Autodesk Inventor part; units mm, degrees
ref_plane "YZ Plane" through (0, 0, 0) normal (1, 0, 0) x (0, 1, 0)
ref_plane "XZ Plane" through (0, 0, 0) normal (0, 1, 0) x (-1, 0, 0)
ref_plane "XY Plane" through (0, 0, 0) normal (0, 0, 1) x (1, 0, 0)
sketch "Sketch1" plane through (0, 0, 0) normal (0, 1, 0) x (-1, 0, 0)
  line L0 (-9, -9) -> (-9, 9)
  line L1 (-9, 9) -> (9, 9)
  line L2 (-8, -8) -> (-8, 8)
  line L3 (-8, 8) -> (8, 8)
  line L4 (0, -8) -> (0, -9)
  line L5 (0, -9) -> (-1, -9)
  line L6 (-8, -8) -> (0, -8)
  line L7 (-9, -9) -> (0, -9)
  line L8 (9, 0) -> (9, 9)
  line L9 (8, 8) -> (8, 1)
  line L10 (9, 0) -> (8, 0)
  line L11 (8, 0) -> (8, 1.1953)
  line L12 (8, 8) -> (8, 9)
  line L13 (-8, 8) -> (-8, 9)
  line L14 (9, 9) -> (8, 9)
  line L15 (-8, 9) -> (-9, 9)
  line L16 (8, 8) -> (7, 8)
  line L17 (7, 8) -> (7, 9)
  line L18 (-8, 8) -> (-7, 8)
  line L19 (-7, 9) -> (-8, 9)
  line L20 (-8, 8) -> (-7, 8)
  line L21 (-7, 8) -> (-7, 9)
  point P0 (0, 0)
  point P1 (0, 11.1675)
  dimension "d4" = 18
  dimension "d5" = 18
  dimension "d10" = 16
  dimension "d11" = 16
  dimension "d33" = 1
  dimension "d62" = 1
  dimension "d63" = 1
extrude "Extrusion1" add sketch "Sketch1" against normal blind 1 contours L0 L1 L13 L2 L6 L4 L5 L7 | L1 L21 L3 L13 | L1 L12 L3 L17 | L1 L8 L10 L11 L9 L12
ref_plane "Work Plane1" through (0, -12, 0) normal (0, -1, 0) x (1, 0, 0)
ref_plane "Work Plane6" through (0, -1, 0) normal (0, -1, 0) x (1, 0, 0)
sketch "Sketch11" plane through (0, -1, 0) normal (0, -1, 0) x (1, 0, 0)
  line L0 (9, 9) -> (-9, 9)
  line L1 (-9, 9) -> (-9, 7)
  line L2 (-9, 0) -> (-9, 9)
  line L3 (-8, 0) -> (-8, 8)
  line L4 (-8, 8) -> (8, 8)
  line L5 (-8, 7) -> (-8, 8)
  line L6 (-8, 8) -> (-7, 8)
  line L7 (-7, 8) -> (-7, 9)
  line L8 (-7, 9) -> (-9, 9)
  line L9 (-9, 7) -> (-8, 7)
  line L10 (9, -9) -> (9, 9)
  line L11 (9, 9) -> (7, 9)
  line L12 (7, 9) -> (7, 8)
  line L13 (7, 8) -> (8, 8)
  line L14 (8, 8) -> (8, 7)
  line L15 (8, 8) -> (8, -8)
  line L16 (9, 7) -> (9, 9)
  line L17 (8, 7) -> (9, 7)
  line L18 (8, -7.9765) -> (8, -6.9765)
  line L19 (8, -6.9765) -> (9, -6.9765)
  line L20 (9, -9) -> (7, -9)
  line L21 (0, -9) -> (9, -9)
  line L22 (8, -8) -> (0, -8)
  line L23 (7, -8) -> (8, -8)
  line L24 (8, -8) -> (7, -8)
  line L25 (7, -9) -> (7, -8)
  point P0 (0, 0)
  dimension "d54" = 2
  dimension "d55" = 1
  dimension "d56" = 2
  dimension "d57" = 1
extrude "Extrusion5" add sketch "Sketch11" along normal blind 10 contours L10 L17 L14 L4 L12 L0 | L7 L4 L3 L9 L1 L0 | L10 L20 L25 L22 L15 L19
sketch "Sketch12" plane through (0, -12, 0) normal (0, -1, 0) x (1, 0, 0)
  line L0 (9, 9) -> (9, -9)
  line L1 (9, 9) -> (9, -9)
  line L2 (9, -9) -> (7.0041, -9)
  line L3 (9, -9) -> (0, -9)
  line L4 (7, -8) -> (7, -9)
  line L5 (7, -8) -> (8, -8)
  line L6 (8, -8) -> (8, 8)
  line L7 (8, -8) -> (8, 8)
  line L8 (8, 8) -> (-8, 8)
  line L9 (8, 8) -> (-8, 8)
  line L10 (-8, 8) -> (-8, 7.0773)
  line L11 (-8, 8) -> (-8, 0)
  line L12 (-8, 7) -> (-9, 7)
  line L13 (-9, 0) -> (-9, 9)
  line L14 (-9, 7) -> (-9, 9)
  line L15 (-9, 9) -> (9, 9)
  line L16 (-9, 9) -> (9, 9)
  point P0 (0, 0)
extrude "Extrusion6" add sketch "Sketch12" against normal blind 1
properties part number "mousecap"
Verification items for the finished model (mm, model axes). A direction names the side the tool comes from. Round coordinates to 2 decimals unless told otherwise and drop trailing zeros. Write each loop counter-clockwise with the first axis right and the second up, starting at its lowest first coordinate (ties: lowest second). Pieces come first, ordered by that corner, then holes.
(1) Section check A-A (z = -3). Enter the section's corners in (x, y).
Returned:
outline: (8, -12) - (9, -12) - (9, -11) - (8, -11) - close; (8, -1) - (9, -1) - (9, 0) - (8, 0) - close
(2) Material ranges on line 1 (Z direction, x = 7.5, y = -1); line 2 (Y direction, x = 8.75, z = 6), recorded low to high.
Returned:
line 1: z = -9 to -8, 8 to 9
line 2: y = -12 to -11, -1 to 0
(3) Depth check by flat-ended pin: pin 1 Ø6 at (x, z) = (3.5, -0.5) entering from +Y; pin 2 Ø0.8 at (x, y) = (-8.5, -0.5) entering from -Z; pin 3 Ø0.8 at (x, y) = (-8.5, -4) entering from -Z; pin 4 Ø1.1 at (y, z) = (-9, -8.5) entering from -X. Enter the tip coordinate at first touch or a pass-through.
Returned:
pin 1: passes through
pin 2: stops at z = 0
pin 3: stops at z = 7
pin 4: stops at x = 7
(4) Section check C-C (z = 6). Enter the section's corners in (x, y), plus the area to 3 significant figures.
Returned:
outline: (-9, -1) - (-8, -1) - (-8, 0) - (-9, 0) - close; (8, -12) - (9, -12) - (9, -11) - (8, -11) - close; (8, -1) - (9, -1) - (9, 0) - (8, 0) - close
area: 3.00 mm2
(5) Section check B-B (y = -3.25). Enter the section's corners in (x, z).
Returned:
outline: (-9, 7) - (-8, 7) - (-8, 8) - (-7, 8) - (-7, 9) - (-9, 9) - close; (7, -9) - (9, -9) - (9, -6.98) - (8, -6.98) - (8, -8) - (7, -8) - close; (7, 8) - (8, 8) - (8, 7) - (9, 7) - (9, 9) - (7, 9) - close
(6) Mould release check, pull along Z, two halves, no side actions. Record for faces 6 (the flat face through (-8, -4.3, 7.3)), 7 (the flat face through (8.5, -11, 0.1)), 8 (the flat face through (7.2, -4.7, -9)): pulls with the +Z half, pulls with the -Z half, needs draft (parallel to the pull), parting line crosses it, or undercut.
Returned:
face 6: needs draft
face 7: undercut
face 8: pulls with the -Z half
(7) Section check D-D (x = 6). Enter the section's corners in (y, z).
Returned:
outline: (-12, 8) - (-11, 8) - (-11, 9) - (-12, 9) - close; (-1, -9) - (0, -9) - (0, -8) - (-1, -8) - close
(8) Access from +Z, -Z, +X, -X, +Y, -Y to the whole of each face (thin tool, end or side, straight path). Record for faces 1 (the flat face through (-8.5, -0.5, 0)), 2 (the flat face through (-8.5, -1, 3.5)), 3 (the flat face through (8, -11.4, 0)), 4 (the flat face through (-0.1, -11, 8.5)), 5 (the flat face through (8.5, -5.9, -6.976)).
Returned:
face 1: -Z, -X, +Y, -Y
face 2: -Z, +X, -X, -Y
face 3: +Y, -Y
face 4: +Z, -Z, +Y
face 5: +X, -X
